Answer from the drawing. Dimensions are ordinates in mm from the lowest x, y and z of the part. A direction names the side the tool comes from. Give positions to 0.01 mm unless a question says otherwise; leave off trailing zeros. Write item = value, one per line.
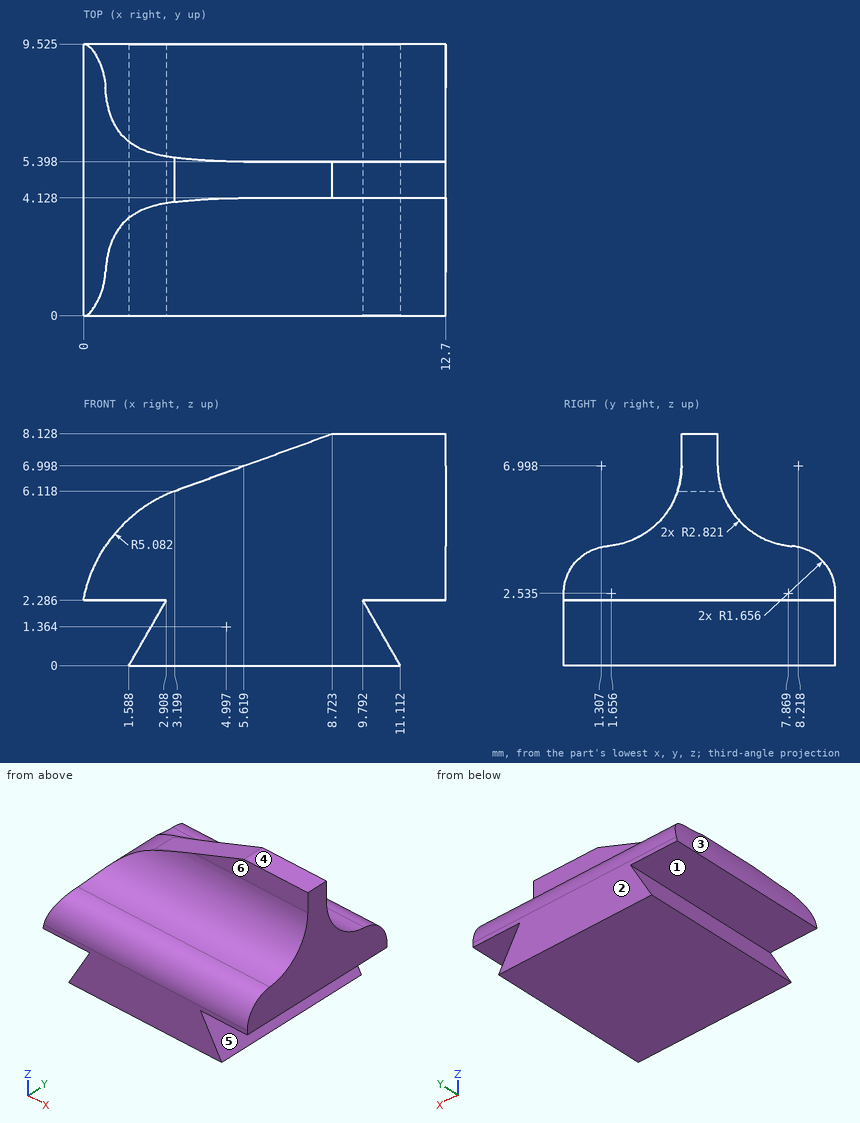
(1) A tool of negligible diameter and unlimited length cuts with its end or side. For the marked faces 4, 5 and 6, from which of +Z, -Z, +X, -X, +Y, -Y can it reach the whole face along a straight path? Write none if from no direction.
Checks:
face_4 = +Z, +X, -X, +Y, -Y
face_5 = +X, +Y, -Y
face_6 = +Z, +X, -X, -Y
(2) Consider L1, parallel to Z at x = 2, y = 7.75 (1 decimal); L2, parallel to Z at x = 10.5, y = 1.5 (1 decimal); L3, parallel to Z at x = 6.5, y = 1.5. Determine where each line is inside the solid, lowest interval first.
Checks:
L1 = 0 to 0.7, 2.3 to 4.2
L2 = 0 to 1.1, 2.3 to 4.2
L3 = 0 to 4.18
(3) For a pull along Z with two mould halves and no side action, classify the marked faces 1, 2 and 3 as released by +Z, released by -Z, zero draft, split by the parting line, or undercut.
Checks:
face_1 = undercut
face_2 = zero draft
face_3 = released by +Z
(4) Given P1, Ø0.6, axis at x = 8.5, z = 8, coming from the -Y side; P2, Ø2, axis at x = 5, z = 7, coming from the -Y side (1 decimal); P3, Ø1, axis at x = 10.5, z = 3.5, coming from the +Y side, each flat-ended and moving along its own axis, determine where each tip first touches the part or whether it passes through.
Checks:
P1 = 4.13
P2 = 3.9
P3 = 9.46
